from build123d import *

# Parameters (mm, degrees)
SKETCH_1_W                      = 89
SKETCH_1_H                      = 70
EXTRUDE_1_DEPTH                 = 12
FILLET_1_R                      = 7.7
CHAMFER_1_SIZE                  = 2.36
SHELL_1_T                       = -2
CUT_EXTRUDE_1_REACH             = 72
SKETCH_2_W                      = 9.92
SKETCH_2_H                      = 7.46
SKETCH_2_W_2                    = 12.93
SKETCH_2_H_2                    = 2.78
CUT_EXTRUDE_2_REACH             = 91
SKETCH_3_W                      = 2.78
SKETCH_3_H                      = 12.93
SKETCH_3_W_2                    = 6.7
SKETCH_3_H_2                    = 17
CUT_EXTRUDE_2_DIRECTION_2_DEPTH = 1
CUT_EXTRUDE_3_REACH             = 91
SKETCH_4_W                      = 2.78
SKETCH_4_H                      = 12.93
SKETCH_5_R                      = 4.5
EXTRUDE_2_DEPTH                 = 10
SKETCH_6_R                      = 1.45
CUT_EXTRUDE_4_DEPTH             = 10.9


with BuildPart() as part:
    # 草圖1 → 填料-伸長1 (new body)
    with BuildSketch(Plane.XY):
        Rectangle(SKETCH_1_W, SKETCH_1_H)
    extrude(amount=EXTRUDE_1_DEPTH)

    # 圓角1
    fillet_1_edges = [part.edges().sort_by_distance(p)[0] for p in [
        (44.5, -35, 6),
        (-44.5, -35, 6),
        (-44.5, 35, 6),
        (44.5, 35, 6),
    ]]
    fillet(fillet_1_edges, radius=FILLET_1_R)

    # 導角1
    chamfer_1_edges = [part.edges().sort_by_distance(p)[0] for p in [
        (44.5, 0, 12),
        (0, -35, 12),
        (0, 35, 12),
        (-44.5, 0, 12),
        (-42.244722215, 32.744722215, 12),
        (-42.244722215, -32.744722215, 12),
        (42.244722215, 32.744722215, 12),
        (42.244722215, -32.744722215, 12),
    ]]
    chamfer(chamfer_1_edges, length=CHAMFER_1_SIZE)

    # 薄殼1
    shell_1_openings = [part.faces().sort_by_distance(p)[0] for p in [
        (0, 0, 0),
    ]]
    offset(amount=SHELL_1_T, openings=shell_1_openings, kind=Kind.INTERSECTION)

    # 草圖2 → 除料-伸長1 (cut, up to next)
    with BuildSketch(Plane(origin=(0, 35, 0), x_dir=(1, 0, 0), z_dir=(0, 1, 0)), mode=Mode.PRIVATE) as cut_extrude_1_sk1:
        with Locations((-11.53, -3.73)):
            Rectangle(SKETCH_2_W, SKETCH_2_H)
    cut_extrude_1_tool1 = extrude(cut_extrude_1_sk1.sketch, amount=-CUT_EXTRUDE_1_REACH, mode=Mode.PRIVATE) & part.part
    add(cut_extrude_1_tool1.solids().sort_by_distance((-11.53, 35, 3.73))[0], mode=Mode.SUBTRACT)
    # 草圖2 → 除料-伸長1 (cut, up to next)
    with BuildSketch(Plane(origin=(0, 35, 0), x_dir=(1, 0, 0), z_dir=(0, 1, 0)), mode=Mode.PRIVATE) as cut_extrude_1_sk2:
        Polygon((-1.5, 0), (-1.5, -4.23), (0.05, -5.777126368), (6.12, -5.777126368), (7.67, -4.23), (7.67, 0), align=None)
    cut_extrude_1_tool2 = extrude(cut_extrude_1_sk2.sketch, amount=-CUT_EXTRUDE_1_REACH, mode=Mode.PRIVATE) & part.part
    add(cut_extrude_1_tool2.solids().sort_by_distance((3.085, 35, 2.77606))[0], mode=Mode.SUBTRACT)
    # 草圖2 → 除料-伸長1 (cut, up to next)
    with BuildSketch(Plane(origin=(0, 35, 0), x_dir=(1, 0, 0), z_dir=(0, 1, 0)), mode=Mode.PRIVATE) as cut_extrude_1_sk3:
        with Locations((19.895, -1.39)):
            Rectangle(SKETCH_2_W_2, SKETCH_2_H_2)
    cut_extrude_1_tool3 = extrude(cut_extrude_1_sk3.sketch, amount=-CUT_EXTRUDE_1_REACH, mode=Mode.PRIVATE) & part.part
    add(cut_extrude_1_tool3.solids().sort_by_distance((19.895, 35, 1.39))[0], mode=Mode.SUBTRACT)

    # 草圖3 → 除料-伸長2 (cut, up to next)
    with BuildSketch(Plane.ZY.offset(44.5), mode=Mode.PRIVATE) as cut_extrude_2_sk1:
        with Locations((1.39, 2.965)):
            Rectangle(SKETCH_3_W, SKETCH_3_H)
    cut_extrude_2_tool1 = extrude(cut_extrude_2_sk1.sketch, amount=-CUT_EXTRUDE_2_REACH, mode=Mode.PRIVATE) & part.part
    add(cut_extrude_2_tool1.solids().sort_by_distance((-44.5, 2.965, 1.39))[0], mode=Mode.SUBTRACT)
    # 草圖3 → 除料-伸長2 (cut, up to next)
    with BuildSketch(Plane.ZY.offset(44.5), mode=Mode.PRIVATE) as cut_extrude_2_sk2:
        with Locations((3.35, -15)):
            Rectangle(SKETCH_3_W_2, SKETCH_3_H_2)
    cut_extrude_2_tool2 = extrude(cut_extrude_2_sk2.sketch, amount=-CUT_EXTRUDE_2_REACH, mode=Mode.PRIVATE) & part.part
    add(cut_extrude_2_tool2.solids().sort_by_distance((-44.5, -15, 3.35))[0], mode=Mode.SUBTRACT)

    # 草圖3 → 除料-伸長2 direction 2 (cut)
    with BuildSketch(Plane.ZY.offset(44.5)):
        with Locations((1.39, 2.965)):
            Rectangle(SKETCH_3_W, SKETCH_3_H)
        with Locations((3.35, -15)):
            Rectangle(SKETCH_3_W_2, SKETCH_3_H_2)
    extrude(amount=CUT_EXTRUDE_2_DIRECTION_2_DEPTH, mode=Mode.SUBTRACT)

    # 草圖4 → 除料-伸長3 (cut, up to next)
    with BuildSketch(Plane(origin=(44.5, 0, 0), x_dir=(0, 0, -1), z_dir=(1, 0, 0)), mode=Mode.PRIVATE) as cut_extrude_3_sk1:
        with Locations((-1.39, 1.535)):
            Rectangle(SKETCH_4_W, SKETCH_4_H)
    cut_extrude_3_tool1 = extrude(cut_extrude_3_sk1.sketch, amount=-CUT_EXTRUDE_3_REACH, mode=Mode.PRIVATE) & part.part
    add(cut_extrude_3_tool1.solids().sort_by_distance((44.5, 1.535, 1.39))[0], mode=Mode.SUBTRACT)

    # 草圖5 → 填料-伸長2 (add)
    with BuildSketch(Plane(origin=(0, 0, 10), x_dir=(-1, 0, 0), z_dir=(0, 0, -1))):
        with Locations((-35.311572875, 25.811572875)):
            Circle(SKETCH_5_R)
        with Locations((35.311572875, 25.811572875)):
            Circle(SKETCH_5_R)
        with Locations((35.311572875, -25.811572875)):
            Circle(SKETCH_5_R)
        with Locations((-35.311572875, -25.811572875)):
            Circle(SKETCH_5_R)
    extrude(amount=EXTRUDE_2_DEPTH)

    # 草圖6 → 除料-伸長4 (cut)
    with BuildSketch(Plane(origin=(0, 0, 0), x_dir=(-1, 0, 0), z_dir=(0, 0, -1))):
        with Locations((-35.311572875, 25.811572875)):
            Circle(SKETCH_6_R)
        with Locations((35.311572875, 25.811572875)):
            Circle(SKETCH_6_R)
        with Locations((35.311572875, -25.811572875)):
            Circle(SKETCH_6_R)
        with Locations((-35.311572875, -25.811572875)):
            Circle(SKETCH_6_R)
    extrude(amount=-CUT_EXTRUDE_4_DEPTH, mode=Mode.SUBTRACT)


solid = part.part
The listing builds one solid part. Answer for the finished solid, in the listing's coordinates (mm). A direction names the side the tool comes from. Round coordinates to 2 decimals unless told otherwise and drop trailing zeros. Loops run counter-clockwise (first coordinate to the right, second up) from the corner with the lowest first, then second, coordinate; pieces in that order, holes last. Notation, with made-up numbers: M 9,31 L 16,31 A17 cw 16,52 Z; hole C 45,81 d6. An arc over 180 degrees is marked long. Write each question's results on one line, items separated by ' | '. Start each with the question number.
1) Find section C-C on z = 1.25. Count the separate pieces of the cut face and the enclosed holes in it, plus the area to 3 significant figures.
2) Straight lines are drawn through the part: probe 1 along X at (y, z) = (3, 8.25); probe 2 along Y at (x, z) = (-36.5, 4.5); probe 3 along X at (y, z) = (-29, 4.5). For each, find the intervals that lie inside material, in ascending order.
3) Find section D-D on y = -22.5. Write down the section's boundary in (x, z).
4) Which of the six approach directions +Z, -Z, +X, -X, +Y, -Y give full straight-line access (tool end or side, diameter ignored) to faces 1 (the cylindrical face through (39.807, 26.009, 5.07)), 2 (the flat face through (-44, -6.5, 3)), 3 (the flat face through (-16.49, 34, 4)), 4 (the flat face through (44.5, 0, 5))?
5) Find section B-B on y = 14. Write down the section's boundary in (x, z), plus the area to 3 significant figures.
6) Each of these flat-tipped pins is pushed along its axis until it touches: pin 1 (2 mm diameter, centred on x = -43.5, z = 2, fed in from -Y); pin 2 (1 mm diameter, centred on y = 34, z = 2, fed in from +X); pin 3 (0.6 mm diameter, centred on y = 34, z = 1.5, fed in from +X). Where does it stop, or does it pass through?
7) Determine the mould class of faces 5 (the flat face through (-6.57, 34, 4)), 6 (the flat face through (-0.52, -33.84, 10.8)), 7 (the flat face through (-42.5, 6, 5)), 8 (the flat face through (44, 1, 2.78)) for opening direction Y: pulls with the +Y half, pulls with the -Y half, needs draft (parallel to the pull), parting line crosses it, or undercut.
8) Find section A-A on x = -26. Write down the section's boundary in (y, z), plus the area to 3 significant figures.
Final values:
1) separate pieces: 10 | enclosed holes: 4 | area: 675 mm²
2) probe 1: -44.5 to -42.5, 42.5 to 44.5 | probe 2: -35 to -33, -30.15 to -26.64, -24.98 to -21.47, 21.47 to 24.98, 26.64 to 30.15, 33 to 35 | probe 3: -44.31 to -42.24, -38.49 to -32.14, 32.14 to 38.49, 42.24 to 44.31
3) outline: M -44.5,6.7 L -42.5,6.7 L -42.5,8.81 L -41.31,10 L -38.36,10 L -38.36,0 L -32.26,0 L -32.26,10 L 32.26,10 L 32.26,0 L 38.36,0 L 38.36,10 L 41.31,10 L 42.5,8.81 L 42.5,0 L 44.5,0 L 44.5,9.64 L 42.14,12 L -42.14,12 L -44.5,9.64 Z
4) face 1: -Z | face 2: -Z, -X | face 3: -Z, +Y | face 4: +Z, -Z, +X, +Y, -Y
5) outline: M -44.5,0 L -42.5,0 L -42.5,8.81 L -41.31,10 L 41.31,10 L 42.5,8.81 L 42.5,0 L 44.5,0 L 44.5,9.64 L 42.14,12 L -42.14,12 L -44.5,9.64 Z | area: 214 mm²
6) pin 1: y = -32.48 | pin 2: x = 41.37 | pin 3: x = 41.08
7) face 5: needs draft | face 6: pulls with the -Y half | face 7: undercut | face 8: undercut
8) outline: M -35,0 L -33,0 L -33,8.81 L -31.81,10 L 31.81,10 L 33,8.81 L 33,0 L 35,0 L 35,9.64 L 32.64,12 L -32.64,12 L -35,9.64 Z | area: 176 mm²
